```python
from build123d import *

# Parameters (mm, degrees)
SKETCH_1_W          = 100
SKETCH_1_H          = 100
EXTRUDE_1_DEPTH     = 15
SKETCH_2_R          = 1.5
CUT_EXTRUDE_1_DEPTH = 143.214626533
SKETCH_3_W          = 50
SKETCH_3_H          = 50
CUT_EXTRUDE_2_DEPTH = 5
SKETCH_4_R          = 5
CUT_EXTRUDE_3_DEPTH = 10
FILLET_1_R          = 5


with BuildPart() as part:
    # 草图1 → 凸台-拉伸1 (new body)
    with BuildSketch(Plane(origin=(0, 0, 0), x_dir=(1, 0, 0), z_dir=(0, 1, 0))):
        with Locations((50, -50)):
            Rectangle(SKETCH_1_W, SKETCH_1_H)
    extrude(amount=EXTRUDE_1_DEPTH)

    # 草图2 → 切除-拉伸1 (cut, through all)
    with BuildSketch(Plane(origin=(0, 15, 0), x_dir=(1, 0, 0), z_dir=(0, 1, 0))):
        with Locations(Location((50, -5, 0), (0, 0, 270))):
            Circle(SKETCH_2_R)
        with Locations(Location((9.585481157, -75, 0), (0, 0, 270))):
            Circle(SKETCH_2_R)
        with Locations(Location((90.414518843, -75, 0), (0, 0, 270))):
            Circle(SKETCH_2_R)
    extrude(amount=-CUT_EXTRUDE_1_DEPTH, mode=Mode.SUBTRACT)

    # 草图3 → 切除-拉伸2 (cut)
    with BuildSketch(Plane(origin=(0, 15, 0), x_dir=(1, 0, 0), z_dir=(0, 1, 0))):
        with Locations((50, -75)):
            Rectangle(SKETCH_3_W, SKETCH_3_H)
    extrude(amount=-CUT_EXTRUDE_2_DEPTH, mode=Mode.SUBTRACT)

    # 草图4 → 切除-拉伸3 (cut)
    with BuildSketch(Plane(origin=(0, 15, 0), x_dir=(1, 0, 0), z_dir=(0, 1, 0))):
        with Locations(Location((10, -10, 0), (0, 0, 270))):
            Circle(SKETCH_4_R)
        with Locations(Location((90, -10, 0), (0, 0, 270))):
            Circle(SKETCH_4_R)
        with Locations(Location((10, -90, 0), (0, 0, 270))):
            Circle(SKETCH_4_R)
        with Locations(Location((90, -90, 0), (0, 0, 270))):
            Circle(SKETCH_4_R)
    extrude(amount=-CUT_EXTRUDE_3_DEPTH, mode=Mode.SUBTRACT)

    # 圆角1
    fillet_1_edges = [part.edges().sort_by_distance(p)[0] for p in [
        (25, 12.5, 50),
        (75, 12.5, 50),
    ]]
    fillet(fillet_1_edges, radius=FILLET_1_R)


solid = part.part
```
Here's how the part is built. I have some questions about the finished solid (model axes, mm). A direction names the side the tool comes from. Coordinates: 2 decimals unless noted, no trailing zeros. Loops run counter-clockwise (first coordinate to the right, second up) from the corner with the lowest first, then second, coordinate; pieces in that order, holes last. Notation, with made-up numbers: (-28.5, -35) - (19.5, -35) arc R22 ccw to (19.5, -17) - close; hole circle Ø2 at (45, -19). An arc over 180 degrees is marked (long way). Return JSON: item names as keys, results as strings. Group by question number.
Item 1: If we section it at C-C on z = 10: Write out the boundary of the cut face in (x, y).
Item 2: If we section it at A-A on z = 75: Write out the boundary of the cut face in (x, y).
Item 3: I need wall thicknesses on line 1 (X direction, y = 9.25, z = 90); line 2 (X direction, y = 4.25, z = 5); line 3 (X direction, y = 5.25, z = 87). Which ranges of each line are inside material? Lowest first, please. Write a range as from..to.
Item 4: If we section it at B-B on x = 50: Write out the boundary of the cut face in (y, z), and give its area (4 significant figures).
Item 5: We'd pull the mould along Z, two halves only. Please class faces 1 (the face through (49, 6, 100)), 2 (the face through (10, 5, 10)), 3 (the face through (49, 7, 0)): +Z half, -Z half, draft (parallel to the pull), parting line (faces both ways), or undercut.
Item 6: Will these pins go through, and if not, where does the flat tip stop? P1, Ø8, axis at x = 90, z = 10, coming from the +Y side; P2, Ø5.5, axis at x = 51, y = 13, coming from the +Z side.
Item 7: On a 3-axis mill with a long thin cutter (end or side, diameter ignored), from which of +Z, -Z, +X, -X, +Y, -Y can I reach the whole of each face in a straight line? I mean faces 4 (the face through (10.04, 7.6, 76.43)), 5 (the face through (90, 5, 10)), 6 (the face through (50, 10, 75)). Say none if no direction works.
Item 8: If we section it at D-D on z = 90: Write out the boundary of the cut face in (x, y).
Calculated:
{
 "1": {"outline": "(0, 0) - (100, 0) - (100, 15) - (95, 15) - (95, 5) - (85, 5) - (85, 15) - (15, 15) - (15, 5) - (5, 5) - (5, 15) - (0, 15) - close"},
 "2": {"outline": "(0, 0) - (8.09, 0) - (8.09, 15) - (0, 15) - close; (11.09, 0) - (88.91, 0) - (88.91, 15) - (75, 15) - (75, 10) - (25, 10) - (25, 15) - (11.09, 15) - close; (91.91, 0) - (100, 0) - (100, 15) - (91.91, 15) - close"},
 "3": {"line 1": "x = 0..5, 15..85, 95..100", "line 2": "x = 0..48.5, 51.5..100", "line 3": "x = 0..6, 14..86, 94..100"},
 "4": {"outline": "(0, 0) - (15, 0) - (15, 3.5) - (0, 3.5) - close; (0, 6.5) - (15, 6.5) - (15, 50) - (10, 50) - (10, 100) - (0, 100) - close", "area": "1,205 mm^2"},
 "5": {"face 1": "+Z half", "face 2": "undercut", "face 3": "-Z half"},
 "6": {"P1": "stops at y = 5", "P2": "stops at z = 50"},
 "7": {"face 4": "+Y, -Y", "face 5": "+Y", "face 6": "+Z, +Y"},
 "8": {"outline": "(0, 0) - (100, 0) - (100, 15) - (95, 15) - (95, 5) - (85, 5) - (85, 15) - (75, 15) - (75, 10) - (25, 10) - (25, 15) - (15, 15) - (15, 5) - (5, 5) - (5, 15) - (0, 15) - close"}
}
